Can you work these out from the model? Positions are in its coordinate system, mm. Give positions to 0.01 mm unless a question says otherwise; leave off trailing zeros. Write each loop counter-clockwise with the first axis right and the second up, starting at its lowest first coordinate (ties: lowest second). Pieces come first, ordered by that corner, then holes.
from build123d import *

# Parameters (mm, degrees)
BOSS_EXTRUDE1_DEPTH = 6
SKETCH2_W           = 6
SKETCH2_H           = 300
CUT_EXTRUDE1_DEPTH  = 6
LPATTERN1_COUNT     = 2
LPATTERN1_PITCH     = 294
CUT_EXTRUDE2_DEPTH  = 6


with BuildPart() as part:
    # Sketch1 → Boss-Extrude1 (new body)
    with BuildSketch(Plane(origin=(0, 0, 0), x_dir=(1, 0, 0), z_dir=(0, 1, 0))):
        Polygon((300, 0), (300, -6), (260, -6), (260, 0), (80, 0), (80, -6), (40, -6), (40, 0), (0, 0), (0, 600), (340, 600), (340, 0), align=None)
    extrude(amount=BOSS_EXTRUDE1_DEPTH)

    # Sketch2 → Cut-Extrude1 (cut)
    with BuildSketch(Plane(origin=(0, 6, 0), x_dir=(1, 0, 0), z_dir=(0, 1, 0))):
        with Locations((23, 150)):
            Rectangle(SKETCH2_W, SKETCH2_H)
    cut_extrude1 = extrude(amount=-CUT_EXTRUDE1_DEPTH, mode=Mode.SUBTRACT)

    # LPattern1: Cut-Extrude1 ×2
    with Locations(*[(i * LPATTERN1_PITCH, 0, 0) for i in range(1, LPATTERN1_COUNT)]):
        add(cut_extrude1, mode=Mode.SUBTRACT)

    # Sketch3 → Cut-Extrude2 (cut)
    with BuildSketch(Plane(origin=(0, 6, 0), x_dir=(1, 0, 0), z_dir=(0, 1, 0))):
        Polygon((70, 600), (270, 600), (270, 588), (257, 588), (257, 594), (83, 594), (83, 588), (70, 588), align=None)
    extrude(amount=-CUT_EXTRUDE2_DEPTH, mode=Mode.SUBTRACT)


solid = part.part
(1) If I drill on L1, parallel to X at y = 1.9, z = -293; L2, parallel to Z at x = 192, y = 4.3; L3, parallel to Z at x = 22.5, y = 0.85, over which ranges is the centre line in solid material (lowest first)?
Returned:
L1: x = 0 to 20, 26 to 314, 320 to 340
L2: z = -594 to 0
L3: z = -600 to -300
(2) Imagine slicing it at B-B, the plane y = 2.45. Write out the boundary of the cut face in (x, z), plus the area to 3 significant figures.
Returned:
outline: (0, -600) - (70, -600) - (70, -588) - (83, -588) - (83, -594) - (257, -594) - (257, -588) - (270, -588) - (270, -600) - (340, -600) - (340, 0) - (320, 0) - (320, -300) - (314, -300) - (314, 0) - (300, 0) - (300, 6) - (260, 6) - (260, 0) - (80, 0) - (80, 6) - (40, 6) - (40, 0) - (26, 0) - (26, -300) - (20, -300) - (20, 0) - (0, 0) - close
area: 200,000 mm2
(3) Imagine slicing it at A-A, the plane z = -153.5. Write out the boundary of the cut face in (x, y).
Returned:
outline: (0, 0) - (20, 0) - (20, 6) - (0, 6) - close; (26, 0) - (314, 0) - (314, 6) - (26, 6) - close; (320, 0) - (340, 0) - (340, 6) - (320, 6) - close
(4) Imagine slicing it at C-C, the plane x = 188.5. Write out the boundary of the cut face in (y, z).
Returned:
outline: (0, -594) - (6, -594) - (6, 0) - (0, 0) - close
(5) Will these pins go through, and if not, where does the flat tip stop? P1, Ø1.8, axis at y = 3.5, z = 3, coming from the -X side; P2, Ø1.8, axis at x = 200.5, y = 4.5, coming from the +Z side; P3, Ø1.8, axis at y = 4.5, z = 1.5, coming from the +X side.
Returned:
P1: stops at x = 40
P2: stops at z = 0
P3: stops at x = 300
